from build123d import *

# Parameters (mm, degrees)
BOSS_EXTRUDE1_DEPTH = 25
BOSS_EXTRUDE2_DEPTH = 18
SKETCH3_W           = 42
SKETCH3_H           = 10
BOSS_EXTRUDE3_DEPTH = 70
CUT_EXTRUDE1_REACH  = 194.188
SKETCH4_R           = 9
SKETCH5_W           = 42
SKETCH5_H           = 12
BOSS_EXTRUDE4_DEPTH = 32
CUT_EXTRUDE2_REACH  = 183.571
SKETCH6_R           = 4


with BuildPart() as part:
    # Sketch1 → Boss-Extrude1 (new body)
    with BuildSketch(Plane(origin=(0, 0, 0), x_dir=(1, 0, 0), z_dir=(0, 1, 0))):
        Polygon((57.307550645, 0), (135.307550645, 0), (135.307550645, 112), (103.307550645, 112), (57.307550645, 89), align=None)
    extrude(amount=-BOSS_EXTRUDE1_DEPTH)

    # Sketch2 → Boss-Extrude2 (add)
    with BuildSketch(Plane.XY):
        Polygon((57.307550645, 0), (127.307550645, 0), (99.307550645, 43), (99.307550645, 53), (57.307550645, 53), align=None)
    extrude(amount=-BOSS_EXTRUDE2_DEPTH)

    # Sketch3 → Boss-Extrude3 (add)
    with BuildSketch(Plane.XY):
        with Locations((78.307550645, 48)):
            Rectangle(SKETCH3_W, SKETCH3_H)
    extrude(amount=-BOSS_EXTRUDE3_DEPTH)

    # Sketch4 → Cut-Extrude1 (cut, up to next)
    with BuildSketch(Plane(origin=(0, 53, 0), x_dir=(1, 0, 0), z_dir=(0, 1, 0)), mode=Mode.PRIVATE) as cut_extrude1_sk1:
        with Locations(Location((78.307550645, 50, 0), (0, 0, 270))):
            Circle(SKETCH4_R)
    cut_extrude1_tool1 = extrude(cut_extrude1_sk1.sketch, amount=-CUT_EXTRUDE1_REACH, mode=Mode.PRIVATE) & part.part
    add(cut_extrude1_tool1.solids().sort_by_distance((78.307551, 53, -50))[0], mode=Mode.SUBTRACT)

    # Sketch5 → Boss-Extrude4 (add)
    with BuildSketch(Plane.ZY.offset(-57.307550645)):
        with Locations((21, 1)):
            Rectangle(SKETCH5_W, SKETCH5_H)
    extrude(amount=-BOSS_EXTRUDE4_DEPTH)

    # Sketch6 → Cut-Extrude2 (cut, up to next)
    with BuildSketch(Plane(origin=(0, 7, 0), x_dir=(1, 0, 0), z_dir=(0, 1, 0)), mode=Mode.PRIVATE) as cut_extrude2_sk1:
        with Locations(Location((67.307550645, -31, 0), (0, 0, 270))):
            Circle(SKETCH6_R)
    cut_extrude2_tool1 = extrude(cut_extrude2_sk1.sketch, amount=-CUT_EXTRUDE2_REACH, mode=Mode.PRIVATE) & part.part
    # Sketch6 → Cut-Extrude2 (cut, up to next)
    with BuildSketch(Plane(origin=(0, 7, 0), x_dir=(1, 0, 0), z_dir=(0, 1, 0)), mode=Mode.PRIVATE) as cut_extrude2_sk2:
        with Locations(Location((77.307550645, -19, 0), (0, 0, 270))):
            Circle(SKETCH6_R)
    cut_extrude2_tool2 = extrude(cut_extrude2_sk2.sketch, amount=-CUT_EXTRUDE2_REACH, mode=Mode.PRIVATE) & part.part
    add(cut_extrude2_tool1.solids().sort_by_distance((67.307551, 7, 31))[0], mode=Mode.SUBTRACT)
    add(cut_extrude2_tool2.solids().sort_by_distance((77.307551, 7, 19))[0], mode=Mode.SUBTRACT)


solid = part.part
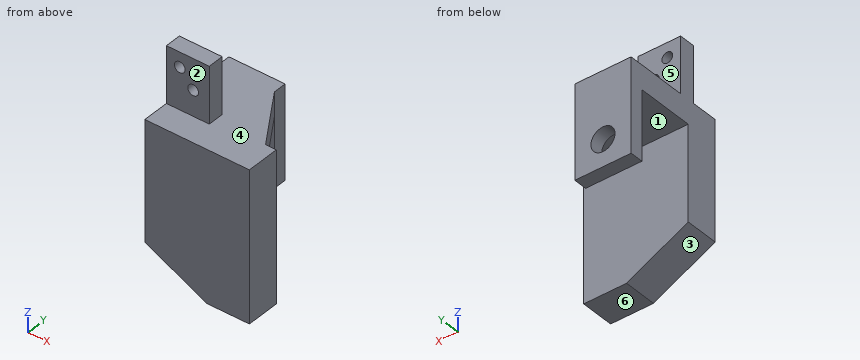
The listing builds one solid part. Answer for the finished solid, in the listing's coordinates (mm). Face numbers are marked on the shaded views. A direction names the side the tool comes from. Round coordinates to 2 decimals unless told otherwise and drop trailing zeros. Write each loop counter-clockwise with the first axis right and the second up, starting at its lowest first coordinate (ties: lowest second). Pieces come first, ordered by that corner, then holes. Notation, with made-up numbers: (15, 1.25) - (33, 1.25) arc R11 ccw to (33, 19.25) - close; hole circle Ø7 at (25, 31.25). An arc over 180 degrees is marked (long way). Use a Markdown table: item, result. Add a question column.
1. The part is cut by section C-C (z = -15). Write down the section's boundary in (x, y).
2. A tool of negligible diameter and unlimited length cuts with its end or side. For the marked faces 4, 5 and 6, from which of +Z, -Z, +X, -X, +Y, -Y can it reach the whole face along a straight path? Write none if from no direction.
3. The part is cut by section D-D (y = -3). Write down the section's boundary in (x, z), and give its area (3 significant figures).
4. Flat-ended cylindrical pins translate along their axes: P1, Ø2, axis at x = 120.5, z = -50.5, coming from the +Y side; P2, Ø3, axis at x = 84.5, y = 46.5, coming from the -Z side; P3, Ø8, axis at x = 107, y = -15.5, coming from the +Z side; P4, Ø6.5, axis at x = 67.31, z = 31, coming from the +Y side. Find the tip coordinate at first contact, or state that the pin passes through.
5. The part is cut by section A-A (z = -50). Write down the section's boundary in (x, y).
6. The part is cut by section B-B (z = 19). Write down the section's boundary in (x, y), and give its area (3 significant figures).
7. Consider line 1 (Y direction, x = 97.5, z = -35); line 2 (X direction, y = 47, z = -50); line 3 (X direction, y = 0, z = 19). Determine where each line is inside the solid, lowest interval first.
8. For a pull along Y with two mould halves and no side action, classify the marked faces 1, 2 and 3 as +Y half, -Y half, draft (parallel to the pull), parting line (faces both ways), or undercut.
Reported:
| question | item | result |
|---|---|---|
| 1 | outline | (57.31, -25) - (135.31, -25) - (135.31, 0) - (127.31, 0) - (99.31, 43) - (99.31, 53) - (57.31, 53) - close |
| 2 | face 4 | +Z, +X |
| 2 | face 5 | +Z, +X, -X, +Y |
| 2 | face 6 | -Z, +X, -X, +Y, -Y |
| 3 | outline | (57.31, -89) - (103.31, -112) - (135.31, -112) - (135.31, 0) - (89.31, 0) - (89.31, 42) - (57.31, 42) - close; hole circle Ø8 at (67.31, 31); hole circle Ø8 at (77.31, 19) |
| 3 | area | 9,450 mm^2 |
| 4 | P1 | y = 0 |
| 4 | P2 | z = -70 |
| 4 | P3 | z = 0 |
| 4 | P4 | through |
| 5 | outline | (57.31, -25) - (135.31, -25) - (135.31, 0) - (57.31, 0) - close; (57.31, 43) - (69.31, 43) - (69.31, 53) - (57.31, 53) - close; (87.31, 43) - (99.31, 43) - (99.31, 53) - (87.31, 53) - close |
| 6 | outline | (57.31, -5) - (73.31, -5) - (73.31, 7) - (57.31, 7) - close; (81.31, -5) - (89.31, -5) - (89.31, 7) - (81.31, 7) - close |
| 6 | area | 288 mm^2 |
| 7 | line 1 | -25 to 0, 43 to 53 |
| 7 | line 2 | 57.31 to 69.31, 87.31 to 99.31 |
| 7 | line 3 | 57.31 to 73.31, 81.31 to 89.31 |
| 8 | face 1 | undercut |
| 8 | face 2 | -Y half |
| 8 | face 3 | draft |
